Geometry: final body of the model. Coordinates: model frame, mm. A direction names the side the tool comes from. Give positions to 0.01 mm unless a question says otherwise; leave off trailing zeros. Loops run counter-clockwise (first coordinate to the right, second up) from the corner with the lowest first, then second, coordinate; pieces in that order, holes last. Notation, with made-up numbers: (38.25, 72) -> (57.25, 72) arc R28 ccw to (57.25, 94) -> close; hole circle Ø10 at (2, -35.75). An arc over 180 degrees is marked (long way). Answer in a Markdown table with one row per item. Add a question column.
from build123d import *

# Parameters (mm, degrees)
F0_W     = 705
F0_H     = 470
F1_DEPTH = 95
F2_T     = -2.54
F4_DEPTH = 505


with BuildPart() as f1:
    # F0 (on Top) → F1 (new body)
    with BuildSketch(Plane.XY):
        Rectangle(F0_W, F0_H)
    extrude(amount=F1_DEPTH)

    # F2
    f2_openings = [f1.faces().sort_by_distance(p)[0] for p in [
        (0, 0, 0),
    ]]
    offset(amount=F2_T, openings=f2_openings)

    # F3 (on face) → F4 (join)
    with BuildSketch(Plane(origin=(0, 0, 0), x_dir=(1, 0, 0), z_dir=(0, 0, -1))):
        Polygon((352.5, 235), (302.5, 235), (302.5, 232.46), (349.96, 232.46), (349.96, 185), (352.5, 185), align=None)
        Polygon((-352.5, 235), (-352.5, 185), (-349.96, 185), (-349.96, 232.46), (-302.5, 232.46), (-302.5, 235), align=None)
        Polygon((-352.5, -185), (-352.5, -235), (-302.5, -235), (-302.5, -232.46), (-349.96, -232.46), (-349.96, -185), align=None)
        Polygon((302.5, -232.46), (302.5, -235), (352.5, -235), (352.5, -185), (349.96, -185), (349.96, -232.46), align=None)
    extrude(amount=F4_DEPTH)


solid = f1.part
(1) Pin query (flat end, axial travel): pin 1 Ø2 at (x, y) = (-123.5, 234) entering from -Z; pin 2 Ø12 at (x, y) = (-104, 88.5) entering from -Z. Return the tip coordinate at first contact, or that it passes through.
(2) Material intervals for line 1 along Y through (x, z) = (-236, 60); line 2 along X through (y, z) = (205.5, -83); line 3 along Z through (x, y) = (149.5, 205.5), sorted ascending. Write a range as from..to.
(3) Draft query along X for faces 1 (the flat face through (24, 232.46, 14)), 2 (the flat face through (352.5, 1, 19)), 3 (the flat face through (-349.96, 33, 14)), 4 (the flat face through (24, 235, 16)). Return one class per face: +X half, -X half, draft (parallel to the pull), parting line (faces both ways), or undercut.
(4) Cut plane C-C on y = -152. Return the cut outline in (x, z).
(5) Cut plane B-B on x = -119. Return the cut outline in (y, z), then the cut area to 3 significant figures.
(6) Reachability of faces 5 (the flat face through (-2, -232.46, 16)), 6 (the flat face through (-352.5, 34, 16)) from +Z, -Z, +X, -X, +Y, -Y: full face, straight path, thin tool, end or side. Return the list, or none.
(7) Cut plane A-A on z = -299. Return the cut outline in (x, y).
Answer list:
| question | item | result |
|---|---|---|
| 1 | pin 1 | stops at z = 0 |
| 1 | pin 2 | stops at z = 92.46 |
| 2 | line 1 | y = -235..-232.46, 232.46..235 |
| 2 | line 2 | x = -352.5..-349.96, 349.96..352.5 |
| 2 | line 3 | z = 92.46..95 |
| 3 | face 1 | undercut |
| 3 | face 2 | +X half |
| 3 | face 3 | undercut |
| 3 | face 4 | draft |
| 4 | outline | (-352.5, 0) -> (-349.96, 0) -> (-349.96, 92.46) -> (349.96, 92.46) -> (349.96, 0) -> (352.5, 0) -> (352.5, 95) -> (-352.5, 95) -> close |
| 5 | outline | (-235, 0) -> (-232.46, 0) -> (-232.46, 92.46) -> (232.46, 92.46) -> (232.46, 0) -> (235, 0) -> (235, 95) -> (-235, 95) -> close |
| 5 | area | 1,660 mm² |
| 6 | face 5 | -Z |
| 6 | face 6 | +Z, -Z, -X, +Y, -Y |
| 7 | outline | (-352.5, -235) -> (-302.5, -235) -> (-302.5, -232.46) -> (-349.96, -232.46) -> (-349.96, -185) -> (-352.5, -185) -> close; (-352.5, 185) -> (-349.96, 185) -> (-349.96, 232.46) -> (-302.5, 232.46) -> (-302.5, 235) -> (-352.5, 235) -> close; (302.5, -235) -> (352.5, -235) -> (352.5, -185) -> (349.96, -185) -> (349.96, -232.46) -> (302.5, -232.46) -> close; (302.5, 232.46) -> (349.96, 232.46) -> (349.96, 185) -> (352.5, 185) -> (352.5, 235) -> (302.5, 235) -> close |
